Input: part model. Units: mm. Frame: model coordinates. Face numbers are marked on the shaded views. A direction names the side the tool comes from. Give positions to 0.01 mm unless a question says otherwise; leave off trailing zeros. Order: outer loops, then holes, each group sorted by start corner. A loop starts at its lowest first (then second) coordinate and runs counter-clockwise, first axis right, second up. Notation, with made-up numbers: (-25.5, 37.25) - (30.5, 37.25) arc R11 ccw to (30.5, 41.25) - close; hole circle Ø10 at (31.25, 11). An arc over 180 degrees is marked (long way). Answer in a Markdown table with one row per item. Add a question column.
1. Section query A-A on y = -10.5. Return loops of the section in (x, z).
2. Section query B-B on y = -13.75. Return loops of the section in (x, z), and give its area (3 significant figures).
3. Access query for the marked faces 1 and 2. Directions: +Z, -Z, +X, -X, +Y, -Y. A direction counts if a zero-diameter tool reaches every point of the face in a straight line with its end or side. Return the directions, or none.
4. Ray query, line 1 (Z direction, x = 0, y = -11.8); line 2 (X direction, y = -11.25, z = 4); line 3 (Z direction, x = 2, y = -11.5). Return the intervals inside material, ascending. Write a range as [from, to].
5. Mould query, pull axis Z, two halves, no side actions, for the marked faces 3 and 4. Classes: released by +Z, released by -Z, zero draft, split by the parting line, or undercut.
6. Contact query for flat-ended pins moving along their axis: pin 1 (2 mm diameter, centred on x = 8.5, z = -2.5, fed in from +Y); pin 2 (4 mm diameter, centred on x = 7.5, y = -9.5, fed in from +Z); pin 3 (1.5 mm diameter, centred on y = -13, z = 8, fed in from +X); pin 4 (5.5 mm diameter, centred on x = 0, z = 0, fed in from -Y). Output: stop coordinate, or through.
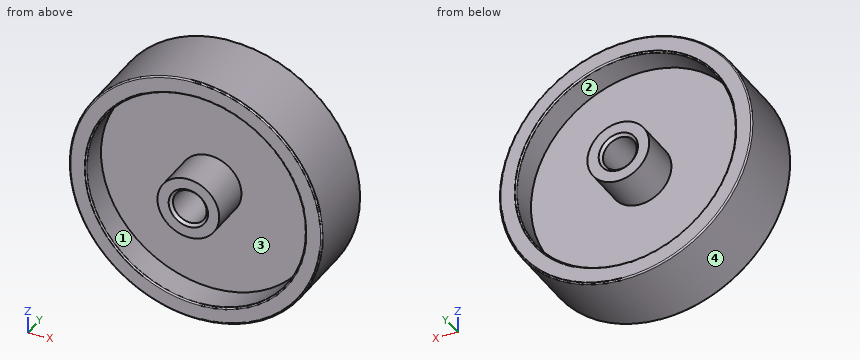
```python
from build123d import *

# Parameters (mm, degrees)
F0_R          = 22.5
F1_DEPTH      = 13
F2_R          = 19.5
F3_DEPTH      = 5
F4_R          = 19.5
F5_DEPTH      = 5
F6_R          = 0.25
F7_R          = 5.5
F7_R_2        = 3
F8_DEPTH      = 7.5
F8_DEPTH_BACK = 10.5
F9_R          = 3
F10_DEPTH     = 25
F11_SIZE      = 0.5


with BuildPart() as f1:
    # F0 (on Front) → F1 (new body)
    with BuildSketch(Plane.XZ):
        Circle(F0_R)
    extrude(amount=F1_DEPTH)

    # F2 (on face) → F3 (cut)
    with BuildSketch(Plane(origin=(0, 0, 0), x_dir=(-1, 0, 0), z_dir=(0, 1, 0))):
        Circle(F2_R)
    extrude(amount=-F3_DEPTH, mode=Mode.SUBTRACT)

    # F4 (on face) → F5 (cut)
    with BuildSketch(Plane.XZ.offset(13)):
        Circle(F4_R)
    extrude(amount=-F5_DEPTH, mode=Mode.SUBTRACT)

    # F6
    f6_edges = [f1.edges().sort_by_distance(p)[0] for p in [
        (-22.5, -13, 0),
        (-22.5, 0, 0),
        (-19.5, -13, 0),
        (19.5, 0, 0),
    ]]
    fillet(f6_edges, radius=F6_R)

    # F7 (on face) → F8 (join, two sides)
    with BuildSketch(Plane.XZ.offset(8)) as f8_sk:
        Circle(F7_R)
        Circle(F7_R_2, mode=Mode.SUBTRACT)
    extrude(amount=F8_DEPTH)
    extrude(f8_sk.sketch, amount=-F8_DEPTH_BACK)

    # F9 (on face) → F10 (cut)
    with BuildSketch(Plane.XZ.offset(15.5)):
        Circle(F9_R)
    extrude(amount=-F10_DEPTH, mode=Mode.SUBTRACT)

    # F11
    f11_edges = [f1.edges().sort_by_distance(p)[0] for p in [
        (-3, -15.5, 0),
        (-3, 2.5, 0),
    ]]
    chamfer(f11_edges, length=F11_SIZE)


solid = f1.part
```
Answer:
| question | item | result |
|---|---|---|
| 1 | outline | circle Ø45 at (0, 0); circle Ø11 at (0, 0); hole circle Ø39 at (0, 0); hole circle Ø6 at (0, 0) |
| 2 | outline | circle Ø11 at (0, 0); hole circle Ø6 at (0, 0) |
| 2 | area | 66.8 mm² |
| 3 | face 1 | -Y |
| 3 | face 2 | +Y |
| 4 | line 1 | z = [-22.5, -19.5], [-5.5, -3], [3, 5.5], [19.5, 22.5] |
| 4 | line 2 | x = [-22.14, -19.09], [-3.77, 3.77], [19.09, 22.14] |
| 4 | line 3 | z = [-22.41, -19.4], [-5.12, -2.24], [2.24, 5.12], [19.4, 22.41] |
| 5 | face 3 | undercut |
| 5 | face 4 | split by the parting line |
| 6 | pin 1 | stops at y = -5 |
| 6 | pin 2 | stops at z = 21.82 |
| 6 | pin 3 | stops at x = 21.29 |
| 6 | pin 4 | passes through |
